Can you work these out from the model? Positions are in its coordinate system, mm. Face numbers are marked on the shaded views. Coordinates: 2 decimals unless noted, no trailing zeros. Order: outer loops, then holes, each group sorted by start corner. A loop starts at its lowest first (then second) coordinate and runs counter-clockwise, first axis right, second up. Notation, with made-up numbers: (49, -11.75) - (100, -11.75) arc R22 cw to (100, 10.25) - close; hole circle Ø7 at (78, 38). An arc over 180 degrees is marked (long way). Return JSON: item names as keys, results as strings. Group by question number.
1) If I drill on line 1 along Y through (x, z) = (43, 27); line 2 along X through (y, z) = (32, 13); line 3 along X through (y, z) = (6, 41), over which ranges is the centre line in solid material (lowest first)?
2) If we mould it in two halves opening along Y, with no side actions, what happens to the marked faces 1, 2 and 3? For each: pulls with the +Y half, pulls with the -Y half, needs draft (parallel to the pull), parting line crosses it, or undercut.
3) Imagine slicing it at A-A (x = 22.5). Write out the boundary of the cut face in (y, z).
4) For pin 1 Ø15 at (y, z) = (36, 36) entering from +X, with a flat end and sliding along its axis, tell me the tip position at first contact or that it passes through.
5) Imagine slicing it at B-B (y = 37). Give the number of separate pieces and of enclosed holes in the cut face, and give its area (3 significant figures).
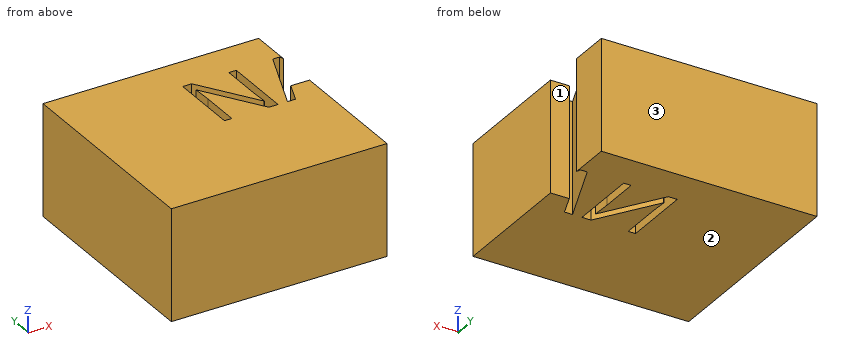
```python
from build123d import *

# Parameters (mm, degrees)
F1_DEPTH = 80


with BuildPart() as f1:
    # F0 (on Top) → F1 (new body)
    with BuildSketch(Plane.XY):
        Polygon((77.5599744916, 46.8204599889), (77.5599744916, 75.9442564845), (-77.5599744916, 75.9442564845), (-77.5599744916, -75.9442564845), (77.5599744916, -75.9442564845), (77.5599744916, 15.7003122036), (64.0222641474, 15.7003122036), (57.9496038182, 0), (52.1362741791, 0), (71.650908618, 49.5753836132), (76.4809427233, 49.5753836132), align=None)
        with BuildLine():
            Line((45.3504544518, 49.3700801502), (45.3504544518, 0))
            Line((45.3504544518, 0), (38.8023545238, 0))
            Line((38.8023545238, 0), (11.8211572957, 41.4280777622))
            Line((11.8211572957, 41.4280777622), (11.5510211601, 41.4280777622))
            add(Edge.make_bspline(
                [(11.5510211601, 41.4280777622), (12.0912934314, 34.1344020999), (12.0912934314, 28.0617417706)],
                knots=[0, 0, 0, 1, 1, 1], degree=2))
            Line((12.0912934314, 28.0617417706), (12.0912934314, 0))
            Line((12.0912934314, 0), (6.7858197274, 0))
            Line((6.7858197274, 0), (6.7858197274, 49.3700801502))
            Line((6.7858197274, 49.3700801502), (13.2690869828, 49.3700801502))
            Line((13.2690869828, 49.3700801502), (40.1854515383, 8.1040840693))
            Line((40.1854515383, 8.1040840693), (40.4555876739, 8.1040840693))
            add(Edge.make_bspline(
                [(40.4555876739, 8.1040840693), (40.3907550014, 9.0117414851), (40.153035202, 13.96063549)],
                knots=[0, 0, 0, 1, 1, 1], degree=2))
            add(Edge.make_bspline(
                [(40.153035202, 13.96063549), (39.9153154026, 18.909529495), (39.9801480752, 21.0382022439)],
                knots=[0, 0, 0, 1, 1, 1], degree=2))
            Line((39.9801480752, 21.0382022439), (39.9801480752, 49.3700801502))
            Line((39.9801480752, 49.3700801502), (45.3504544518, 49.3700801502))
        make_face(mode=Mode.SUBTRACT)
    extrude(amount=F1_DEPTH)


solid = f1.part
```
Calculated:
{
 "1": {"line 1": "-75.94 to 0, 49.37 to 75.94", "line 2": "-77.56 to 6.79, 12.04 to 17.96, 24.6 to 39.98, 45.35 to 64.73", "line 3": "-77.56 to 6.79, 12.09 to 34.89, 45.35 to 54.5, 60.27 to 77.56"},
 "2": {"face 1": "undercut", "face 2": "needs draft", "face 3": "pulls with the +Y half"},
 "3": {"outline": "(-75.94, 0) - (25.03, 0) - (25.03, 80) - (-75.94, 80) - close; (35.22, 0) - (75.94, 0) - (75.94, 80) - (35.22, 80) - close"},
 "4": {"pin 1": "x = 69.26"},
 "5": {"separate pieces": "4", "enclosed holes": "0", "area": "10,200 mm2"}
}
